from build123d import *

# Parameters (mm, degrees)
BOSS_EXTRUDE1_DEPTH = 3
CUT_EXTRUDE1_DEPTH  = 3
SKETCH3_R           = 1
CUT_EXTRUDE2_DEPTH  = 3


with BuildPart() as part:
    # Sketch1 → Boss-Extrude1 (new body)
    with BuildSketch(Plane.XY):
        with BuildLine():
            Line((15, 0), (45, 0))
            Line((45, 0), (45, -3))
            Line((45, -3), (60, -3))
            Line((60, -3), (60, 0))
            Line((60, 0), (60, 70))
            ThreePointArc((60, 70), (57.071067812, 77.071067812), (50, 80))
            Line((50, 80), (10, 80))
            ThreePointArc((10, 80), (2.928932188, 77.071067812), (0, 70))
            Line((0, 70), (0, 0))
            Line((0, 0), (0, -3))
            Line((0, -3), (15, -3))
            Line((15, -3), (15, 0))
        make_face()
    extrude(amount=BOSS_EXTRUDE1_DEPTH)

    # Sketch2 → Cut-Extrude1 (cut)
    with BuildSketch(Plane.XY.offset(3)):
        with BuildLine():
            Line((29.19049781, 12.081147466), (17.107164477, 37.322032883))
            Line((17.107164477, 37.322032883), (17.107164477, 17.497814133))
            add(Edge.make_bspline(
                [(17.107164477, 17.497814133), (17.106856563, 17.267704948), (17.106272319, 16.831089584), (17.143554032, 16.210481556), (17.183991208, 15.655960439), (17.251147223, 15.170009562), (17.322412489, 14.747387769), (17.428594053, 14.398396218), (17.538951634, 14.108390436), (17.644805439, 13.95466925), (17.693101977, 13.884532883)],
                knots=[0, 0, 0, 0, 1.48973486, 2.826663046, 4.025252461, 5.088590954, 6.003687083, 6.795186099, 7.45029523, 8, 8, 8, 8], degree=3))
            add(Edge.make_bspline(
                [(17.693101977, 13.884532883), (17.840346266, 13.73471353), (18.140195748, 13.429620165), (18.742251873, 13.122863505), (19.450963165, 12.941254282), (19.961816932, 12.923746203), (20.232164477, 12.9144808)],
                knots=[0, 0, 0, 0, 0.893460505, 1.819450328, 2.846037184, 4, 4, 4, 4], degree=3))
            Line((20.232164477, 12.9144808), (21.273831144, 12.9144808))
            Line((21.273831144, 12.9144808), (21.273831144, 12.081147466))
            Line((21.273831144, 12.081147466), (10.857164477, 12.081147466))
            Line((10.857164477, 12.081147466), (10.857164477, 12.9144808))
            Line((10.857164477, 12.9144808), (11.898831144, 12.9144808))
            add(Edge.make_bspline(
                [(11.898831144, 12.9144808), (12.048825145, 12.917755098), (12.339180303, 12.924093413), (12.757070795, 12.986186233), (13.143145766, 13.072376691), (13.494447303, 13.206491265), (13.814309401, 13.373094257), (14.09832336, 13.583510491), (14.341505484, 13.83600194), (14.479050655, 14.023925059), (14.548570727, 14.118907883)],
                knots=[0, 0, 0, 0, 1.182386838, 2.288838982, 3.326958154, 4.296765023, 5.246416275, 6.164047556, 7.072046332, 8, 8, 8, 8], degree=3))
            add(Edge.make_bspline(
                [(14.548570727, 14.118907883), (14.587376699, 14.189630143), (14.672804719, 14.345319134), (14.767344621, 14.622115391), (14.841068835, 14.959225842), (14.914129522, 15.351610192), (14.965303143, 15.806218983), (14.991936983, 16.317094802), (15.023349157, 16.887654031), (15.023664816, 17.28725487), (15.023831144, 17.497814133)],
                knots=[0, 0, 0, 0, 0.561580455, 1.236271222, 2.028879402, 2.966584022, 4.017422664, 5.2149421, 6.532486222, 8, 8, 8, 8], degree=3))
            Line((15.023831144, 17.497814133), (15.023831144, 36.6644808))
            add(Edge.make_bspline(
                [(15.023831144, 36.6644808), (15.02055328, 36.988166413), (15.014467946, 37.589086891), (14.928768358, 38.415621701), (14.807342688, 39.104328259), (14.655869132, 39.495898491), (14.587633227, 39.6722933)],
                knots=[0, 0, 0, 0, 1.269100049, 2.356076937, 3.259444487, 4, 4, 4, 4], degree=3))
            add(Edge.make_bspline(
                [(14.587633227, 39.6722933), (14.530456066, 39.780881674), (14.412829383, 40.004273146), (14.162927878, 40.302631077), (13.844654076, 40.567219507), (13.462503112, 40.813691306), (12.979301958, 41.020762409), (12.378141387, 41.15502888), (11.658107064, 41.237530633), (11.137387273, 41.244216283), (10.857164477, 41.247814133)],
                knots=[0, 0, 0, 0, 0.685675889, 1.410594349, 2.160436148, 2.996293973, 3.94870651, 5.086176952, 6.431940446, 8, 8, 8, 8], degree=3))
            Line((10.857164477, 41.247814133), (10.857164477, 42.081147466))
            Line((10.857164477, 42.081147466), (19.398831144, 42.081147466))
            Line((19.398831144, 42.081147466), (30.55768531, 18.7738558))
            Line((30.55768531, 18.7738558), (41.716539477, 42.081147466))
            Line((41.716539477, 42.081147466), (50.023831144, 42.081147466))
            Line((50.023831144, 42.081147466), (50.023831144, 41.247814133))
            Line((50.023831144, 41.247814133), (49.001695727, 41.247814133))
            add(Edge.make_bspline(
                [(49.001695727, 41.247814133), (48.849510318, 41.244694592), (48.556943778, 41.238697479), (48.135006283, 41.175164667), (47.746219832, 41.091107105), (47.393177435, 40.955606693), (47.072846278, 40.789567822), (46.789193443, 40.576638492), (46.539300059, 40.328607353), (46.401580276, 40.138732081), (46.332424894, 40.04338705)],
                knots=[0, 0, 0, 0, 1.192663738, 2.292818382, 3.341598875, 4.305885976, 5.250132179, 6.162540657, 7.077327887, 8, 8, 8, 8], degree=3))
            add(Edge.make_bspline(
                [(46.332424894, 40.04338705), (46.293618922, 39.97266479), (46.208190902, 39.816975798), (46.113651, 39.540179542), (46.039926786, 39.20306909), (45.966866099, 38.810684741), (45.915692478, 38.35607595), (45.889058638, 37.845200131), (45.857646464, 37.274640902), (45.857330805, 36.875040062), (45.857164477, 36.6644808)],
                knots=[0, 0, 0, 0, 0.561580455, 1.236271222, 2.028879402, 2.966584022, 4.017422664, 5.2149421, 6.532486222, 8, 8, 8, 8], degree=3))
            Line((45.857164477, 36.6644808), (45.857164477, 17.497814133))
            add(Edge.make_bspline(
                [(45.857164477, 17.497814133), (45.856887283, 17.267711351), (45.856361328, 16.831108136), (45.893253556, 16.210418928), (45.934944838, 15.656159203), (45.99825562, 15.168982955), (46.081396816, 14.748408827), (46.183028471, 14.396778863), (46.302123125, 14.10774347), (46.412242488, 13.95460789), (46.462633227, 13.884532883)],
                knots=[0, 0, 0, 0, 1.486776415, 2.821049613, 4.017258766, 5.078485589, 5.994452933, 6.784380121, 7.443731031, 8, 8, 8, 8], degree=3))
            add(Edge.make_bspline(
                [(46.462633227, 13.884532883), (46.609751164, 13.734446531), (46.910693137, 13.427432419), (47.515250463, 13.125895229), (48.222218515, 12.940045729), (48.731216692, 12.923351845), (49.001695727, 12.9144808)],
                knots=[0, 0, 0, 0, 0.893634595, 1.828003868, 2.845812335, 4, 4, 4, 4], degree=3))
            Line((49.001695727, 12.9144808), (50.023831144, 12.9144808))
            Line((50.023831144, 12.9144808), (50.023831144, 12.081147466))
            Line((50.023831144, 12.081147466), (37.523831144, 12.081147466))
            Line((37.523831144, 12.081147466), (37.523831144, 12.9144808))
            Line((37.523831144, 12.9144808), (38.56549781, 12.9144808))
            add(Edge.make_bspline(
                [(38.56549781, 12.9144808), (38.717654175, 12.917695974), (39.010164878, 12.923876936), (39.430396151, 12.985823667), (39.817804477, 13.074062693), (40.171351147, 13.203103474), (40.488581605, 13.375227668), (40.771335549, 13.583465527), (41.01486323, 13.834271299), (41.148211479, 14.02369587), (41.215237394, 14.118907883)],
                knots=[0, 0, 0, 0, 1.198333024, 2.303717216, 3.340834392, 4.325725627, 5.259386468, 6.176132048, 7.08325442, 8, 8, 8, 8], degree=3))
            add(Edge.make_bspline(
                [(41.215237394, 14.118907883), (41.254043366, 14.189630143), (41.339471385, 14.345319134), (41.434011288, 14.622115391), (41.507735502, 14.959225842), (41.580796189, 15.351610192), (41.631969809, 15.806218983), (41.658603649, 16.317094802), (41.690015823, 16.887654031), (41.690331482, 17.28725487), (41.69049781, 17.497814133)],
                knots=[0, 0, 0, 0, 0.561580455, 1.236271222, 2.028879402, 2.966584022, 4.017422664, 5.2149421, 6.532486222, 8, 8, 8, 8], degree=3))
            Line((41.69049781, 17.497814133), (41.69049781, 37.322032883))
            Line((41.69049781, 37.322032883), (29.607164477, 12.081147466))
            Line((29.607164477, 12.081147466), (29.19049781, 12.081147466))
        make_face()
    extrude(amount=-CUT_EXTRUDE1_DEPTH, mode=Mode.SUBTRACT)

    # Sketch3 → Cut-Extrude2 (cut)
    with BuildSketch(Plane.XY.offset(3)):
        with Locations((15, 64.377519573)):
            Circle(SKETCH3_R)
        with Locations((45, 64.377519573)):
            Circle(SKETCH3_R)
        with Locations((23, 64.377519573)):
            Circle(SKETCH3_R)
        with Locations((37, 64.377519573)):
            Circle(SKETCH3_R)
    extrude(amount=-CUT_EXTRUDE2_DEPTH, mode=Mode.SUBTRACT)


solid = part.part
Source: CAD feature listing. Evaluate the final solid. Frame: model axes, mm. A direction names the side the tool comes from. Round coordinates to 2 decimals unless told otherwise and drop trailing zeros. Loops run counter-clockwise (first coordinate to the right, second up) from the corner with the lowest first, then second, coordinate; pieces in that order, holes last.
Q1. Access query for faces 4 (the face through (15, -2, 1)), 5 (the face through (23.233, 24.525, 1.521)), 6 (the face through (52, -3, 1)). Directions: +Z, -Z, +X, -X, +Y, -Y. A direction counts if a zero-diameter tool reaches every point of the face in a straight line with its end or side. Return the directions, or none.
Q2. First-contact query: P1, Ø1.1, axis at x = 38, z = 1, coming from the -Y side. Flat tip, straight axial feed; report the tip coordinate or a pass-through.
Q3. Mould query, pull axis Y, two halves, no side actions, for faces 1 (the face through (3.01, 77.15, 1.48)), 2 (the face through (30, 39, 0)), 3 (the face through (41.69, 27, 2)). Classes: pulls with the +Y half, pulls with the -Y half, needs draft (parallel to the pull), parting line crosses it, or undercut.
Q4. Section B-B, the plane y = 26. Return loops of the section in (x, z).
Q5. Section C-C, the plane z = 0.5. State how many separate pieces and enclosed holes the cut face has, plus the area to 3 significant figures.
Q6. Ray query, line 1 (Y direction, x = 43.5, z = 2.55); line 2 (X direction, y = 38, z = 1.1); line 3 (Y direction, x = 37, z = 1.45). Return the intervals inside material, ascending.
Q7. Section A-A, the plane x = 43. Return loops of the section in (y, z).
Solutions:
1. face 4: +Z, -Z, -Y
1. face 5: +Z, -Z
1. face 6: +Z, -Z, +X, -X, -Y
2. P1: stops at y = 0
3. face 1: pulls with the +Y half
3. face 2: needs draft
3. face 3: undercut
4. outline: (0, 0) - (15.02, 0) - (15.02, 3) - (0, 3) - close; (17.11, 0) - (22.53, 0) - (22.53, 3) - (17.11, 3) - close; (27.1, 0) - (34.02, 0) - (34.02, 3) - (27.1, 3) - close; (36.27, 0) - (41.69, 0) - (41.69, 3) - (36.27, 3) - close; (45.86, 0) - (60, 0) - (60, 3) - (45.86, 3) - close
5. separate pieces: 1
5. enclosed holes: 5
5. area: 4,440 mm2
6. line 1: y = 0 to 12.08, 42.08 to 80
6. line 2: x = 0 to 14.97, 21.35 to 39.76, 45.9 to 60
6. line 3: y = 0 to 27.52, 32.23 to 63.38, 65.38 to 80
7. outline: (0, 0) - (12.08, 0) - (12.08, 3) - (0, 3) - close; (42.08, 0) - (80, 0) - (80, 3) - (42.08, 3) - close
